```python
from build123d import *

# Parameters (mm, degrees)
SKETCH1_W           = 91
SKETCH1_H           = 57
BOSS_EXTRUDE1_DEPTH = 2
FILLET1_R           = 2
SKETCH2_W           = 91
SKETCH2_H           = 57
SKETCH2_W_2         = 87
SKETCH2_H_2         = 53
BOSS_EXTRUDE6_DEPTH = 15
FILLET2_R           = 2
SKETCH13_W          = 5
SKETCH13_H          = 5
BOSS_EXTRUDE7_DEPTH = 3


with BuildPart() as part:
    # Sketch1 → Boss-Extrude1 (new body)
    with BuildSketch(Plane(origin=(0, 0, 0), x_dir=(1, 0, 0), z_dir=(0, 1, 0))):
        with Locations((45.5, 28.5)):
            Rectangle(SKETCH1_W, SKETCH1_H)
    extrude(amount=BOSS_EXTRUDE1_DEPTH)

    # Fillet1
    fillet1_edges = [part.edges().sort_by_distance(p)[0] for p in [
        (0, 1, -57),
        (91, 1, -57),
        (91, 1, 0),
        (0, 1, 0),
    ]]
    fillet(fillet1_edges, radius=FILLET1_R)

    # Sketch2 → Boss-Extrude6 (add)
    with BuildSketch(Plane(origin=(0, 2, 0), x_dir=(1, 0, 0), z_dir=(0, 1, 0))):
        with Locations((45.5, 28.5)):
            Rectangle(SKETCH2_W, SKETCH2_H)
        with Locations((45.5, 28.5)):
            Rectangle(SKETCH2_W_2, SKETCH2_H_2, mode=Mode.SUBTRACT)
    extrude(amount=BOSS_EXTRUDE6_DEPTH)

    # Fillet2
    fillet2_edges = [part.edges().sort_by_distance(p)[0] for p in [
        (0, 9.5, -57),
        (91, 9.5, -57),
        (91, 9.5, 0),
        (0, 9.5, 0),
    ]]
    fillet(fillet2_edges, radius=FILLET2_R)

    # Sketch13 → Boss-Extrude7 (add)
    with BuildSketch(Plane(origin=(0, 2, 0), x_dir=(1, 0, 0), z_dir=(0, 1, 0))):
        with Locations((4.5, 52.5)):
            Rectangle(SKETCH13_W, SKETCH13_H)
        with Locations((4.5, 4.5)):
            Rectangle(SKETCH13_W, SKETCH13_H)
        with Locations((59.5, 52.5)):
            Rectangle(SKETCH13_W, SKETCH13_H)
        with Locations((59.5, 4.5)):
            Rectangle(SKETCH13_W, SKETCH13_H)
    extrude(amount=BOSS_EXTRUDE7_DEPTH)


solid = part.part
```
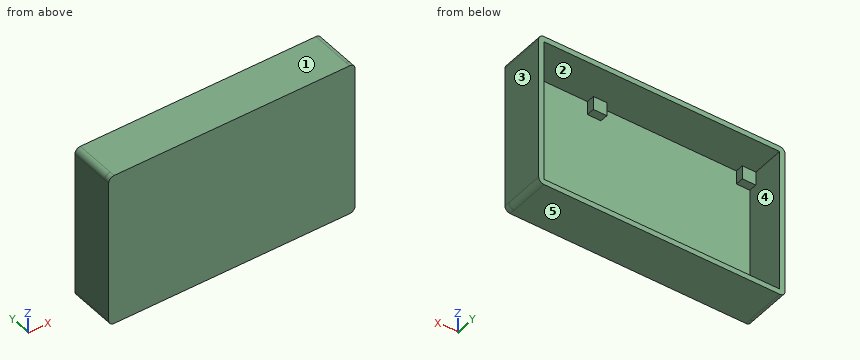
Work out the finished part from the listing and answer in its coordinate system (mm). Face numbers are marked on the shaded views. A direction names the side the tool comes from. Round coordinates to 2 decimals unless told otherwise and drop trailing zeros. Loops run counter-clockwise (first coordinate to the right, second up) from the corner with the lowest first, then second, coordinate; pieces in that order, holes last.
(1) The part is cut by section A-A, the plane y = 3. Give the vertices of the cut face in (x, z).
Computed values:
outline: (0, -55) arc R2 ccw to (2, -57) - (89, -57) arc R2 ccw to (91, -55) - (91, -2) arc R2 ccw to (89, 0) - (2, 0) arc R2 ccw to (0, -2) - close; hole (2, -50) - (7, -50) - (7, -55) - (57, -55) - (57, -50) - (62, -50) - (62, -55) - (89, -55) - (89, -2) - (62, -2) - (62, -7) - (57, -7) - (57, -2) - (7, -2) - (7, -7) - (2, -7) - close
(2) Find the intervals of material crossed by L1, parallel to Z at x = 13.5, y = 15.5; L2, parallel to X at y = 12.5, z = -43; L3, parallel to Y at x = 34, z = -16.5, in increasing order.
Computed values:
L1: z = -57 to -55, -2 to 0
L2: x = 0 to 2, 89 to 91
L3: y = 0 to 2
(3) Each of these flat-tipped pins is pushed along its axis until it touches: P1, Ø5, axis at x = 35.5, z = -12, coming from the +Y side; P2, Ø10, axis at x = 39, z = -42, coming from the -Y side; P3, Ø1.5, axis at x = 59.5, z = -53, coming from the +Y side. Where does it stop, or does it pass through?
Computed values:
P1: stops at y = 2
P2: stops at y = 0
P3: stops at y = 5
(4) The part is cut by section C-C, the plane z = -4.5. Give the vertices of the cut face in (x, y).
Computed values:
outline: (0, 0) - (91, 0) - (91, 17) - (89, 17) - (89, 2) - (62, 2) - (62, 5) - (57, 5) - (57, 2) - (7, 2) - (7, 5) - (2, 5) - (2, 17) - (0, 17) - close
(5) The mould has two halves that part along Z. Classify the marked faces 1, 2 and 3: pulls with the +Z half, pulls with the -Z half, needs draft (parallel to the pull), parting line crosses it, or undercut.
Computed values:
face 1: pulls with the +Z half
face 2: undercut
face 3: needs draft
(6) The part is cut by section B-B, the plane x = 39.5. Give the vertices of the cut face in (y, z), and give its area (3 significant figures).
Computed values:
outline: (0, -57) - (17, -57) - (17, -55) - (2, -55) - (2, -2) - (17, -2) - (17, 0) - (0, 0) - close
area: 174 mm2
(7) For the marked faces 4 and 5, determine the directions among +Z, -Z, +X, -X, +Y, -Y from which every point of the face is accessible in a straight line to the end or side of a thin tool.
Computed values:
face 4: +Y
face 5: -Z, +X, -X, +Y, -Y
(8) The part is cut by section D-D, the plane y = 12.5. Give the vertices of the cut face in (x, z).
Computed values:
outline: (0, -55) arc R2 ccw to (2, -57) - (89, -57) arc R2 ccw to (91, -55) - (91, -2) arc R2 ccw to (89, 0) - (2, 0) arc R2 ccw to (0, -2) - close; hole (2, -55) - (89, -55) - (89, -2) - (2, -2) - close
